Could you check a few things on this model? Use its own coordinates, in mm. A direction names the side the tool comes from. Round coordinates to 2 decimals unless told otherwise and drop trailing zeros. Loops run counter-clockwise (first coordinate to the right, second up) from the corner with the lowest first, then second, coordinate; pieces in that order, holes last.
from build123d import *

# Parameters (mm, degrees)
SKETCH_1_W                     = 125
SKETCH_1_H                     = 85
EXTRUDE_1_DEPTH                = 5
SKETCH_2_W                     = 15
SKETCH_2_H                     = 15
CUT_EXTRUDE_1_DEPTH            = 5
PATTERN_LINEAR_1_COUNT         = 6
PATTERN_LINEAR_1_PITCH         = 20
PATTERN_LINEAR_1_COUNT_DIR2    = 4
PATTERN_LINEAR_1_PITCH_DIR2    = 20
EXTRUDE_START                  = -5
SKETCH_3_W                     = 5
SKETCH_3_H                     = 10
EXTRUDE_2_DEPTH                = 15
PATTERN_LINEAR_2_COUNT         = 2
PATTERN_LINEAR_2_PITCH         = 69
CUT_EXTRUDE_START              = -15
SKETCH_5_W                     = 5.5
SKETCH_5_H                     = 5.5
CUT_EXTRUDE_3_DEPTH            = 125
SKETCH_9_R                     = 0.1
EXTRUDE_3_DEPTH                = 1
PATTERN_CIRCULAR_1_OUTLINE_W   = 4.5
PATTERN_CIRCULAR_1_OUTLINE_H   = 5
PATTERN_CIRCULAR_1_OUTLINE_W_2 = 5
PATTERN_CIRCULAR_1_DEPTH       = 10
PATTERN_START                  = 5.5
PATTERN_CIRCULAR_1_2_OUTLINE_W = 5.5
PATTERN_CIRCULAR_1_2_OUTLINE_H = 5
PATTERN_CIRCULAR_1_2_DEPTH     = 4.5


# Read off the part's stored shape, not the designer's step: 阵列(圆周)1
with BuildPart() as part:
    # 草图1 → 凸台-拉伸1 (new body)
    with BuildSketch(Plane(origin=(0, 0, 0), x_dir=(1, 0, 0), z_dir=(0, 1, 0))):
        with Locations((62.5, -42.5)):
            Rectangle(SKETCH_1_W, SKETCH_1_H)
    extrude(amount=EXTRUDE_1_DEPTH)

    # 草图2 → 切除-拉伸1 (cut)
    with BuildSketch(Plane(origin=(0, 5, 0), x_dir=(1, 0, 0), z_dir=(0, 1, 0))):
        with Locations((12.5, -12.5)):
            Rectangle(SKETCH_2_W, SKETCH_2_H)
    cut_extrude_1 = extrude(amount=-CUT_EXTRUDE_1_DEPTH, mode=Mode.SUBTRACT)

    # 阵列(线性)1: Cut-Extrude 1 6 × 4
    with Locations(*[(i * PATTERN_LINEAR_1_PITCH, 0, j * PATTERN_LINEAR_1_PITCH_DIR2) for i in range(PATTERN_LINEAR_1_COUNT) for j in range(PATTERN_LINEAR_1_COUNT_DIR2) if (i, j) != (0, 0)]):
        add(cut_extrude_1, mode=Mode.SUBTRACT)

    # 草图3 → 凸台-拉伸2 (add)
    with BuildSketch(Plane(origin=(125, 0, 0), x_dir=(0, 0, -1), z_dir=(1, 0, 0)).offset(EXTRUDE_START)):
        with Locations((-8, 5)):
            Rectangle(SKETCH_3_W, SKETCH_3_H)
    extrude_2 = extrude(amount=EXTRUDE_2_DEPTH)

    # 阵列(线性)2: 凸台-拉伸2 ×2
    with Locations(*[(0, 0, i * PATTERN_LINEAR_2_PITCH) for i in range(1, PATTERN_LINEAR_2_COUNT)]):
        add(extrude_2)

    # 草图5 → 切除-拉伸3 (cut)
    with BuildSketch(Plane.XY.offset(10.5).offset(CUT_EXTRUDE_START)):
        with Locations((127.75, 2.75)):
            Rectangle(SKETCH_5_W, SKETCH_5_H)
    extrude(amount=CUT_EXTRUDE_3_DEPTH, mode=Mode.SUBTRACT)

    # 草图9 → 凸台-拉伸3 (add)
    with BuildSketch(Plane(origin=(0, 5, 0), x_dir=(1, 0, 0), z_dir=(0, 1, 0))):
        with Locations(Location((62.5, -42.5, 0), (0, 0, 270))):
            Circle(SKETCH_9_R)
    extrude(amount=EXTRUDE_3_DEPTH)

    # 阵列(圆周)1 outline → 阵列(圆周)1 (add)
    with BuildSketch(Plane(origin=(0, 0, 0), x_dir=(1, 0, 0), z_dir=(0, 1, 0))):
        with Locations((-7.75, -77)):
            Rectangle(PATTERN_CIRCULAR_1_OUTLINE_W, PATTERN_CIRCULAR_1_OUTLINE_H)
        with Locations((2.5, -8)):
            Rectangle(PATTERN_CIRCULAR_1_OUTLINE_W_2, PATTERN_CIRCULAR_1_OUTLINE_H)
        with Locations((2.5, -77)):
            Rectangle(PATTERN_CIRCULAR_1_OUTLINE_W_2, PATTERN_CIRCULAR_1_OUTLINE_H)
        with Locations((-7.75, -8)):
            Rectangle(PATTERN_CIRCULAR_1_OUTLINE_W, PATTERN_CIRCULAR_1_OUTLINE_H)
    extrude(amount=PATTERN_CIRCULAR_1_DEPTH)

    # Pattern Circular 1 2 outline → Pattern Circular 1 2 (add)
    with BuildSketch(Plane(origin=(0, 0, 0), x_dir=(1, 0, 0), z_dir=(0, 1, 0)).offset(PATTERN_START)):
        with Locations((-2.75, -8)):
            Rectangle(PATTERN_CIRCULAR_1_2_OUTLINE_W, PATTERN_CIRCULAR_1_2_OUTLINE_H)
        with Locations((-2.75, -77)):
            Rectangle(PATTERN_CIRCULAR_1_2_OUTLINE_W, PATTERN_CIRCULAR_1_2_OUTLINE_H)
    extrude(amount=PATTERN_CIRCULAR_1_2_DEPTH)


solid = part.part
Item 1: If we section it at A-A, the plane x = 73: Please give me the cut outline in (y, z), then the cut area to 3 significant figures.
Results list:
outline: (0, 0) - (5, 0) - (5, 5) - (0, 5) - close; (0, 20) - (5, 20) - (5, 25) - (0, 25) - close; (0, 40) - (5, 40) - (5, 45) - (0, 45) - close; (0, 60) - (5, 60) - (5, 65) - (0, 65) - close; (0, 80) - (5, 80) - (5, 85) - (0, 85) - close
area: 125 mm2
Item 2: Will these pins go through, and if not, where does the flat tip stop? pin 1 (6 mm diameter, centred on x = 74, z = 56, fed in from +Y); pin 2 (5.5 mm diameter, centred on y = 2.5, z = 32.5, fed in from +X); pin 3 (4 mm diameter, centred on y = 3.5, z = 42.5, fed in from -X); pin 4 (3 mm diameter, centred on x = -6, y = 5, fed in from +Z).
Results list:
pin 1: passes through
pin 2: stops at x = 125
pin 3: stops at x = 0
pin 4: stops at z = 79.5
Item 3: If we section it at B-B, the plane y = 3.25: Count the separate pieces of the cut face and the enclosed holes in it, then the cut area to 4 significant figures.
Results list:
separate pieces: 5
enclosed holes: 24
area: 5,315 mm2
Item 4: If we section it at D-D, the plane x = 122: Please give me the cut outline in (y, z).
Results list:
outline: (0, 0) - (5, 0) - (5, 5.5) - (10, 5.5) - (10, 10.5) - (5, 10.5) - (5, 74.5) - (10, 74.5) - (10, 79.5) - (5, 79.5) - (5, 85) - (0, 85) - close
Item 5: If we section it at C-C, the plane z = 47: Please give me the cut outline in (x, y), then the cut area to 3 significant figures.
Results list:
outline: (0, 0) - (5, 0) - (5, 5) - (0, 5) - close; (20, 0) - (25, 0) - (25, 5) - (20, 5) - close; (40, 0) - (45, 0) - (45, 5) - (40, 5) - close; (60, 0) - (65, 0) - (65, 5) - (60, 5) - close; (80, 0) - (85, 0) - (85, 5) - (80, 5) - close; (100, 0) - (105, 0) - (105, 5) - (100, 5) - close; (120, 0) - (125, 0) - (125, 5) - (120, 5) - close
area: 175 mm2
Item 6: We'd pull the mould along X, two halves only. Please class faces 4 (the flat face through (129, 6, 74.5)), 5 (the flat face through (5, 4, 74)): released by +X, released by -X, zero draft, split by the parting line, or undercut.
Results list:
face 4: zero draft
face 5: undercut
Item 7: If I drill on line 1 along Z through (x, y) = (17, 2); line 2 along Z through (x, y) = (126.5, 5.75); line 3 along Y through (x, z) = (2, 31.5), over which ranges is the centre line in solid material (lowest first)?
Results list:
line 1: z = 0 to 5, 20 to 25, 40 to 45, 60 to 65, 80 to 85
line 2: z = 5.5 to 10.5, 74.5 to 79.5
line 3: y = 0 to 5
Item 8: For faces 1 (the flat face through (-4, 6, 10.5)), 2 (the flat face through (100, 3, 13)), 3 (the flat face through (-3, 5.5, 77)), which set-ups out of +Z, -Z, +X, -X, +Y, -Y let a thin tool reach every point of the face, with its end or its side?
Results list:
face 1: -X, +Y
face 2: +Y, -Y
face 3: +Z, -Z, -Y
